```python
from build123d import *

# Parameters (mm, degrees)
F0_W     = 70
F0_H     = 34
F1_DEPTH = 1
F2_R     = 5


with BuildPart() as f1:
    # F0 (on Top) → F1 (new body)
    with BuildSketch(Plane.XY):
        Rectangle(F0_W, F0_H)
        with BuildLine():
            ThreePointArc((-30, 10.5), (-31.0606601718, 13.0606601718), (-28.5, 12))
            Line((-28.5, 12), (28.5, 12))
            ThreePointArc((28.5, 12), (30, 13.5), (31.5, 12))
            ThreePointArc((31.5, 12), (31.0606601718, 10.9393398282), (30, 10.5))
            Line((30, 10.5), (30, -10.5))
            ThreePointArc((30, -10.5), (31.0606601718, -10.9393398282), (31.5, -12))
            ThreePointArc((31.5, -12), (30, -13.5), (28.5, -12))
            Line((28.5, -12), (-28.5, -12))
            ThreePointArc((-28.5, -12), (-31.0606601718, -13.0606601718), (-30, -10.5))
            Line((-30, -10.5), (-30, 10.5))
        make_face(mode=Mode.SUBTRACT)
        with BuildLine():
            Line((28.5, 12), (-28.5, 12))
            ThreePointArc((-28.5, 12), (-28.9393398282, 10.9393398282), (-30, 10.5))
            Line((-30, 10.5), (-30, -10.5))
            ThreePointArc((-30, -10.5), (-28.9393398282, -10.9393398282), (-28.5, -12))
            Line((-28.5, -12), (28.5, -12))
            ThreePointArc((28.5, -12), (28.9393398282, -10.9393398282), (30, -10.5))
            Line((30, -10.5), (30, 10.5))
            ThreePointArc((30, 10.5), (28.9393398282, 10.9393398282), (28.5, 12))
        make_face()
    extrude(amount=F1_DEPTH)

    # F2
    f2_edges = [f1.edges().sort_by_distance(p)[0] for p in [
        (-35, -17, 0.5),
        (-35, 17, 0.5),
        (35, 17, 0.5),
        (35, -17, 0.5),
    ]]
    fillet(f2_edges, radius=F2_R)


solid = f1.part
```
The model under review builds one solid part; all positions refer to its coordinate system, in mm. Give positions to 0.01 mm unless a question says otherwise; leave off trailing zeros. Write each loop counter-clockwise with the first axis right and the second up, starting at its lowest first coordinate (ties: lowest second). Pieces come first, ordered by that corner, then holes.
(1) To check wall thickness, follow L1, parallel to Y at x = -30, z = 0.3; L2, parallel to X at y = -12, z = 0.45; L3, parallel to X at y = 15, z = 0.65. State the ranges of each line that lie inside material, in increasing order.
(2) For P1, Ø1.8, axis at x = -30, y = -12, coming from the +Z side, flat-tipped, find the tip position at first contact; note if it passes through.
(3) Consider section A-A, the plane z = 0.35. Give the boundary of the cut face in (x, y).
Returned:
1. L1: y = -17 to -13.5, -10.5 to 10.5, 13.5 to 17
1. L2: x = -35 to -31.5, -28.5 to 28.5, 31.5 to 35
1. L3: x = -34 to 34
2. P1: passes through
3. outline: (-35, -12) arc R5 ccw to (-30, -17) - (30, -17) arc R5 ccw to (35, -12) - (35, 12) arc R5 ccw to (30, 17) - (-30, 17) arc R5 ccw to (-35, 12) - close; hole circle Ø3 at (-30, -12); hole circle Ø3 at (-30, 12); hole circle Ø3 at (30, -12); hole circle Ø3 at (30, 12)
